```python
from build123d import *

# Parameters (mm, degrees)
F0_R     = 27.5
F1_DEPTH = 7.5
F2_R     = 7.49999
F3_DEPTH = 2.5
F4_DEPTH = 5


# Not quite as in the source:
# - a fillet or chamfer is up to 0.001 mm smaller than in the source, because OpenCascade refuses the exact size


with BuildPart() as f1:
    # F0 (on Front) → F1 (new body, symmetric)
    with BuildSketch(Plane.XZ):
        Circle(F0_R)
        Polygon((1.325, 0.7649891067), (1.325, 0), (1.325, -0.7649891067), (0.6624999921, -1.1474836645), (0, -1.5299782134), (-0.6624999921, -1.1474836645), (-1.325, -0.7649891067), (-1.325, 0), (-1.325, 0.7649891067), (-0.6624999921, 1.1474836645), (0, 1.5299782134), (0.6624999921, 1.1474836645), align=None, mode=Mode.SUBTRACT)
    extrude(amount=F1_DEPTH, both=True)

    # F2 (radius 7.5 in the source; OpenCascade refuses exactly that, so slightly less here)
    f2_edges = [f1.edges().sort_by_distance(p)[0] for p in [
        (-27.5, -7.5, 0),
        (-27.5, 7.5, 0),
    ]]
    fillet(f2_edges, radius=F2_R)

    # F3 (cut, symmetric): a face of the model
    f3_faces = [f1.faces().sort_by_distance(p)[0] for p in [
        (-19.4343242922, -7.5, 0),
    ]]
    extrude(f3_faces, amount=F3_DEPTH, both=True, mode=Mode.SUBTRACT)

    # F4 (cut): a face of the model
    f4_faces = [f1.faces().sort_by_distance(p)[0] for p in [
        (-19.4343242922, 7.5, 0),
    ]]
    extrude(f4_faces, amount=-F4_DEPTH, mode=Mode.SUBTRACT)


solid = f1.part
```
The model under review builds one solid part; all positions refer to its coordinate system, in mm. A direction names the side the tool comes from. Give positions to 0.01 mm unless a question says otherwise; leave off trailing zeros. Answer in a Markdown table with one row per item.
Item 1: For P1, Ø5, axis at x = -10, z = 13.5, coming from the +Y side; P2, Ø2, axis at y = 4.5, z = -17.5, coming from the +X side; P3, Ø24, axis at x = 0, z = 0, coming from the -Y side; P4, Ø1.7, axis at y = -0.5, z = 0, coming from the +X side, all flat-tipped, find the tip position at first contact; note any pin that passes through.
Check sheet entries:
| item | result |
|---|---|
| P1 | y = 2.5 |
| P2 | x = 20.46 |
| P3 | y = -5 |
| P4 | x = 27.5 |
Item 2: Tool access review of faces 1 (the face through (-4.336, -6.268, -19.524)), 2 (the face through (1.325, -1, 0)), 3 (the face through (0, 2.5, -4)): name each direction out of +Z, -Z, +X, -X, +Y, -Y from which nothing blocks a thin tool from reaching the whole face with its end or side.
Check sheet entries:
| item | result |
|---|---|
| face 1 | -Y |
| face 2 | +Y, -Y |
| face 3 | +Y |
Item 3: For line 1 along Y through (x, z) = (-8.5, -3); line 2 along X through (y, z) = (3, 15); line 3 along Z through (x, y) = (0, 3.6), list the stretches that pass through material, from the lowest coordinate up.
Check sheet entries:
| item | result |
|---|---|
| line 1 | -5 to 2.5 |
| line 2 | -22.3 to -13.23, 13.23 to 22.3 |
| line 3 | -26.58 to -20, 20 to 26.58 |
